```python
from build123d import *

# Parameters (mm, degrees)
SKETCH1_W                                = 65
SKETCH1_H                                = 38.1
SKETCH1_W_2                              = 41
SKETCH1_H_2                              = 21
BOSS_EXTRUDE1_DEPTH                      = 8
SKETCH2_W                                = 65
SKETCH2_H                                = 38.1
SKETCH2_W_2                              = 59
SKETCH2_H_2                              = 26.1
BOSS_EXTRUDE2_DEPTH                      = 15
F_5_32_0_15625_DIAMETER_HOLE1_D          = 3.96875
F_3_0MM_DOWEL_HOLE1_D                    = 3
F_3_0MM_DOWEL_HOLE1_DEPTH                = 6
CUT_EXTRUDE1_DEPTH                       = 2.25
MIRROR2_AT_THE_SECOND_PLANE_COPY_1_DEPTH = 2.25
SKETCH9_W                                = 6
SKETCH9_H                                = 2
CUT_EXTRUDE2_DEPTH                       = 8


with BuildPart() as part:
    # Sketch1 → Boss-Extrude1 (new body)
    with BuildSketch(Plane(origin=(0, 0, 0), x_dir=(0, 0, -1), z_dir=(1, 0, 0))):
        Rectangle(SKETCH1_W, SKETCH1_H)
        Rectangle(SKETCH1_W_2, SKETCH1_H_2, mode=Mode.SUBTRACT)
    extrude(amount=BOSS_EXTRUDE1_DEPTH)

    # Sketch2 → Boss-Extrude2 (add)
    with BuildSketch(Plane(origin=(8, 0, 0), x_dir=(0, 0, -1), z_dir=(1, 0, 0))):
        Rectangle(SKETCH2_W, SKETCH2_H)
        Rectangle(SKETCH2_W_2, SKETCH2_H_2, mode=Mode.SUBTRACT)
    extrude(amount=BOSS_EXTRUDE2_DEPTH)

    # 5/32 (0.15625) Diameter Hole1 (through all)
    with Locations(Plane.ZY):
        with Locations((-23.60854322, 5.122882485), (-23.749, -5.08), (23.749, -5.08), (23.749, 5.08)):
            Hole(F_5_32_0_15625_DIAMETER_HOLE1_D / 2)

    # Ø3.0mm Dowel Hole1
    with Locations(Plane(origin=(0, -13.05, 0), x_dir=(1, 0, 0), z_dir=(0, 1, 0))):
        with Locations((11.5, 25), (11.5, -25)):
            f_3_0mm_dowel_hole1 = Hole(F_3_0MM_DOWEL_HOLE1_D / 2, depth=F_3_0MM_DOWEL_HOLE1_DEPTH)

    # Mirror1: Ø3.0mm Dowel Hole1 across plane
    add(f_3_0mm_dowel_hole1.mirror(Plane.ZX), mode=Mode.SUBTRACT)

    # Sketch7 → Cut-Extrude1 (cut)
    with BuildSketch(Plane(origin=(0, -13.05, 0), x_dir=(1, 0, 0), z_dir=(0, 1, 0))):
        Polygon((8.775, -26.573279484), (11.5, -28.146558967), (14.225, -26.573279484), (14.225, -23.426720516), (11.5, -21.853441033), (8.775, -23.426720516), align=None)
    cut_extrude1 = extrude(amount=-CUT_EXTRUDE1_DEPTH, mode=Mode.SUBTRACT)

    # Mirror2: Cut-Extrude1 across plane
    add(cut_extrude1.mirror(Plane.ZX), mode=Mode.SUBTRACT)

    # Mirror2 at the second plane: Cut-Extrude1 across plane
    add(cut_extrude1.mirror(Plane.XY), mode=Mode.SUBTRACT)

    # Mirror2 at the second plane copy 1 sketc → Mirror2 at the second plane copy 1 (cut)
    with BuildSketch(Plane.XZ.offset(-13.05)):
        Polygon((8.775, -26.573279484), (11.5, -28.146558967), (14.225, -26.573279484), (14.225, -23.426720516), (11.5, -21.853441033), (8.775, -23.426720516), align=None)
    extrude(amount=-MIRROR2_AT_THE_SECOND_PLANE_COPY_1_DEPTH, mode=Mode.SUBTRACT)

    # Sketch9 → Cut-Extrude2 (cut)
    with BuildSketch(Plane.ZY):
        with Locations((-23.5, 0)):
            Rectangle(SKETCH9_W, SKETCH9_H)
        with Locations((23.5, 0)):
            Rectangle(SKETCH9_W, SKETCH9_H)
    extrude(amount=-CUT_EXTRUDE2_DEPTH, mode=Mode.SUBTRACT)


solid = part.part
```
Geometry: final body of the model. Coordinates: model frame, mm. A direction names the side the tool comes from. Coordinates: 2 decimals unless noted, no trailing zeros. Loops run counter-clockwise (first coordinate to the right, second up) from the corner with the lowest first, then second, coordinate; pieces in that order, holes last. Notation, with made-up numbers: M 55,25 L 113,25 A17 ccw 113,33 Z; hole C -14.75,59.25 d10. An arc over 180 degrees is marked long. Put each result on its own line as item: value.
(1) First-contact query: pin 1 (1.5 mm diameter, centred on y = -10.5, z = -20.5, fed in from +X); pin 2 (1.8 mm diameter, centred on y = -14.5, z = 24.5, fed in from -X). Flat tips, straight axial feed; report the tip coordinate or a pass-through.
Answer sheet:
pin 1: stops at x = 8
pin 2: stops at x = 0
(2) Cut plane A-A on y = -5.08. Return the cut outline in (x, z), then the cut area to 4 significant figures.
Answer sheet:
outline: M 0,-32.5 L 23,-32.5 L 23,-29.5 L 8,-29.5 L 8,-25.73 L 0,-25.73 Z; M 0,-21.76 L 8,-21.76 L 8,-20.5 L 0,-20.5 Z; M 0,20.5 L 8,20.5 L 8,21.76 L 0,21.76 Z; M 0,25.73 L 8,25.73 L 8,29.5 L 23,29.5 L 23,32.5 L 0,32.5 Z
area: 218.5 mm^2
(3) Material intervals for probe 1 along Z at (x, y) = (11.5, 16.2); probe 2 along Y at (x, z) = (9.25, 1); probe 3 along Y at (x, z) = (3, -18.5), sorted ascending.
Answer sheet:
probe 1: z = -32.5 to -26.5, -23.5 to 23.5, 26.5 to 32.5
probe 2: y = -19.05 to -13.05, 13.05 to 19.05
probe 3: y = -19.05 to -10.5, 10.5 to 19.05
(4) Cut plane D-D on z = -19.5. Return the cut outline in (x, y), then the cut area to 3 significant figures.
Answer sheet:
outline: M 0,-19.05 L 23,-19.05 L 23,-13.05 L 8,-13.05 L 8,-10.5 L 0,-10.5 Z; M 0,10.5 L 8,10.5 L 8,13.05 L 23,13.05 L 23,19.05 L 0,19.05 Z
area: 317 mm^2
(5) Cut plane B-B on x = 19.75. Return the cut outline in (y, z), then the cut area to 3 significant figures.
Answer sheet:
outline: M -19.05,-32.5 L 19.05,-32.5 L 19.05,32.5 L -19.05,32.5 Z; hole M -13.05,-29.5 L 13.05,-29.5 L 13.05,29.5 L -13.05,29.5 Z
area: 937 mm^2
(6) Access query for faces 4 (the face through (15, 0, 29.5)), 5 (the face through (12.843, 14.159, 27.371)), 6 (the face through (4, 1, -24)). Directions: +Z, -Z, +X, -X, +Y, -Y. A direction counts if a zero-diameter tool reaches every point of the face in a straight line with its end or side. Return the directions, or none.
Answer sheet:
face 4: +X
face 5: none
face 6: +X, -X
(7) Draft query along Y for faces 1 (the face through (11.695, -17.201, -26.487)), 2 (the face through (11, -19.05, 0)), 3 (the face through (15, 0, -29.5)). Return one class per face: pulls with the +Y half, pulls with the -Y half, needs draft (parallel to the pull), parting line crosses it, or undercut.
Answer sheet:
face 1: needs draft
face 2: pulls with the -Y half
face 3: undercut
(8) Cut plane C-C on y = 8. Return the cut outline in (x, z).
Answer sheet:
outline: M 0,-32.5 L 23,-32.5 L 23,-29.5 L 8,-29.5 L 8,-20.5 L 0,-20.5 Z; M 0,20.5 L 8,20.5 L 8,29.5 L 23,29.5 L 23,32.5 L 0,32.5 Z
